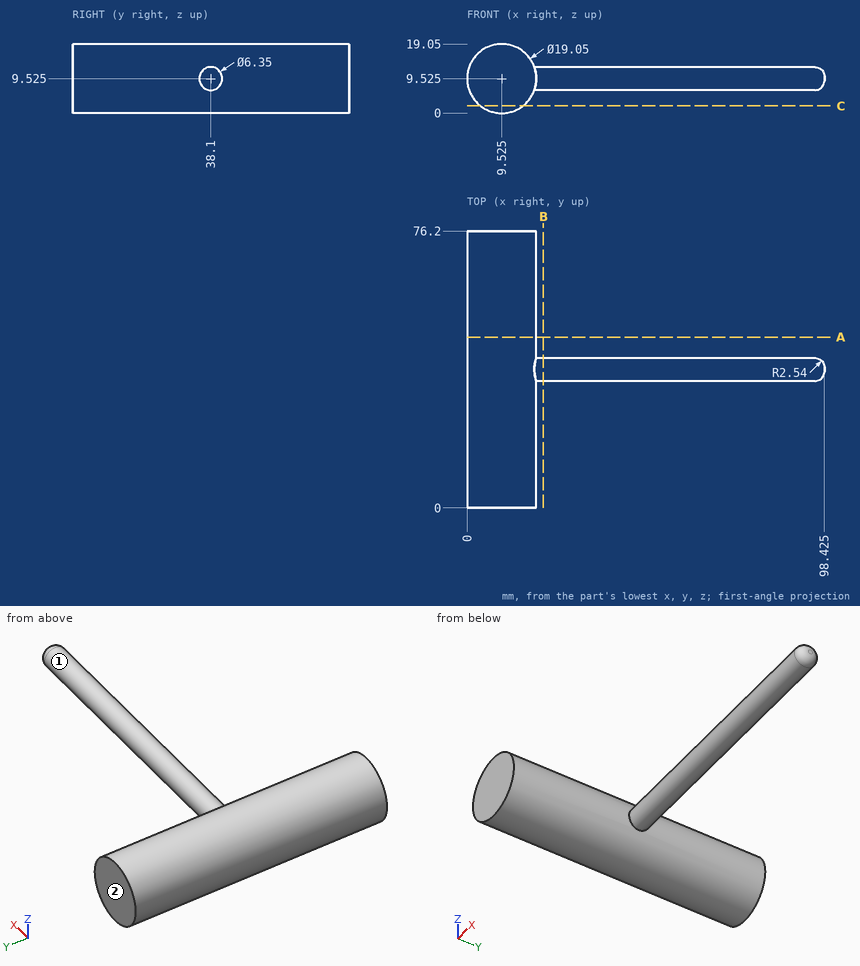
The drawing under review shows one solid part. Ordinate dimensions are in mm from its lowest x, y, z. A direction names the side the tool comes from. Round coordinates to 2 decimals unless told otherwise and drop trailing zeros. Write each loop counter-clockwise with the first axis right and the second up, starting at its lowest first coordinate (ties: lowest second). Pieces come first, ordered by that corner, then holes. Notation, with made-up numbers: (-14.75, -35.5) -> (31.25, -35.5) arc R30 cw to (31.25, -12.5) -> close; hole circle Ø4 at (83, 76). An arc over 180 degrees is marked (long way). One line per question, with ' | ' between items.
(1) Wall thickness on line 1 (Y direction, x = 57, z = 12); line 2 (X direction, y = 72.5, z = 5); line 3 (X direction, y = 63, z = 1.75): over which ranges is each line inside the solid? List them lowest first. Write a range as [from, to].
Result sheet:
line 1: [36.11, 40.09] | line 2: [1.14, 17.91] | line 3: [4.02, 15.03]
(2) Machinability: for the marked faces 1 and 2, which of the approach directions +Z, -Z, +X, -X, +Y, -Y give a long, thin tool a straight path to every point of the face, cutting with its end or side? Answer none if there is none.
Result sheet:
face 1: +X | face 2: +Z, -Z, +X, -X, +Y
(3) Take a section at A-A, the plane y = 47. State the section outline as (x, z) points (3 decimals), and give its area (3 significant figures).
Result sheet:
outline: circle Ø19.05 at (9.525, 9.525) | area: 285 mm2
(4) Take a section at C-C, the plane z = 2. State the section outline as (x, y) points.
Result sheet:
outline: (3.69, 0) -> (15.36, 0) -> (15.36, 76.2) -> (3.69, 76.2) -> close
(5) Insertion check: P1, Ø3, axis at x = 29.5, z = 13.5, coming from the +Y side; P2, Ø5, axis at x = 78, z = 11, coming from the +Y side (3 decimals); P3, Ø8, axis at x = 36.5, z = 3.5, coming from the -Y side. Each pin has a flat end and moves straight along its axis. Give the tip position at first contact, or say it passes through.
Result sheet:
P1: y = 40.09 | P2: y = 41.275 | P3: y = 35.65
(6) Take a section at B-B, the plane x = 21. State the section outline as (y, z) points (3 decimals), and give its area (3 significant figures).
Result sheet:
outline: circle Ø6.35 at (38.1, 9.525) | area: 31.7 mm2
